```python
from build123d import *

# Parameters (mm, degrees)
SKETCH1_R           = 1.6
BOSS_EXTRUDE1_DEPTH = 27
CUT_EXTRUDE1_REACH  = 138.335
SKETCH2_R           = 2.1
CUT_EXTRUDE2_REACH  = 155.174
SKETCH3_R           = 1.7
SKETCH3_3_R         = 3
SKETCH3_3_R_2       = 1.7
CUT_EXTRUDE3_DEPTH  = 3
SKETCH4_R           = 3
CUT_EXTRUDE4_DEPTH  = 8
BOSS_EXTRUDE2_START = -27
BOSS_EXTRUDE2_DEPTH = 27
FILLET1_R           = 10


with BuildPart() as part:
    # Sketch1 → Boss-Extrude1 (new body)
    with BuildSketch(Plane.XY.offset(10)):
        with BuildLine():
            Line((-25.534872354, -37.053613776), (50.619597549, -89.534180987))
            ThreePointArc((50.619597549, -89.534180987), (54.361803385, -90.334528675), (57.573873786, -88.254320829))
            Line((57.573873786, -88.254320829), (58.227827632, -87.305369414))
            ThreePointArc((58.227827632, -87.305369414), (59.02817532, -83.563163578), (56.947967474, -80.351093178))
            Line((56.947967474, -80.351093178), (-21.854778729, -26.045511066))
            ThreePointArc((-21.854778729, -26.045511066), (-26.045511066, 21.854778729), (21.854778729, 26.045511066))
            Line((21.854778729, 26.045511066), (89.019290298, -42.129978983))
            ThreePointArc((89.019290298, -42.129978983), (92.543786433, -43.620813626), (96.090160837, -42.182797794))
            Line((96.090160837, -42.182797794), (96.911137653, -41.373995292))
            ThreePointArc((96.911137653, -41.373995292), (98.401972296, -37.849499157), (96.963956464, -34.303124754))
            Line((96.963956464, -34.303124754), (32.056602073, 31.581232775))
            ThreePointArc((32.056602073, 31.581232775), (-34.47199994, 28.925442436), (-25.534872354, -37.053613776))
        make_face()
        with Locations((90.17973297, -37.494440018)):
            Circle(SKETCH1_R, mode=Mode.SUBTRACT)
        with Locations((68.973861607, -16.273907044)):
            Circle(SKETCH1_R, mode=Mode.SUBTRACT)
        with Locations((47.767990244, 4.946625931)):
            Circle(SKETCH1_R, mode=Mode.SUBTRACT)
        with Locations((18.75, 32.475952642)):
            Circle(SKETCH1_R, mode=Mode.SUBTRACT)
        with Locations((-6.511806663, 36.930290738)):
            Circle(SKETCH1_R, mode=Mode.SUBTRACT)
        with Locations((-28.726666617, 24.104535363)):
            Circle(SKETCH1_R, mode=Mode.SUBTRACT)
        with Locations((-37.5, 0)):
            Circle(SKETCH1_R, mode=Mode.SUBTRACT)
        with Locations((-28.726666617, -24.104535363)):
            Circle(SKETCH1_R, mode=Mode.SUBTRACT)
        with Locations((3.423348889, -47.901259716)):
            Circle(SKETCH1_R, mode=Mode.SUBTRACT)
        with Locations((28.003855203, -65.100059364)):
            Circle(SKETCH1_R, mode=Mode.SUBTRACT)
        with Locations((52.584361518, -82.298859012)):
            Circle(SKETCH1_R, mode=Mode.SUBTRACT)
    extrude(amount=BOSS_EXTRUDE1_DEPTH)

    # Sketch2 → Cut-Extrude1 (cut, up to next)
    with BuildSketch(Plane.XY.offset(37), mode=Mode.PRIVATE) as cut_extrude1_sk1:
        with Locations((52.584361518, -82.298859012)):
            Circle(SKETCH2_R)
    cut_extrude1_tool1 = extrude(cut_extrude1_sk1.sketch, amount=-CUT_EXTRUDE1_REACH, mode=Mode.PRIVATE) & part.part
    # Sketch2 → Cut-Extrude1 (cut, up to next)
    with BuildSketch(Plane.XY.offset(37), mode=Mode.PRIVATE) as cut_extrude1_sk2:
        with Locations((28.003855203, -65.100059364)):
            Circle(SKETCH2_R)
    cut_extrude1_tool2 = extrude(cut_extrude1_sk2.sketch, amount=-CUT_EXTRUDE1_REACH, mode=Mode.PRIVATE) & part.part
    # Sketch2 → Cut-Extrude1 (cut, up to next)
    with BuildSketch(Plane.XY.offset(37), mode=Mode.PRIVATE) as cut_extrude1_sk3:
        with Locations((3.423348889, -47.901259716)):
            Circle(SKETCH2_R)
    cut_extrude1_tool3 = extrude(cut_extrude1_sk3.sketch, amount=-CUT_EXTRUDE1_REACH, mode=Mode.PRIVATE) & part.part
    # Sketch2 → Cut-Extrude1 (cut, up to next)
    with BuildSketch(Plane.XY.offset(37), mode=Mode.PRIVATE) as cut_extrude1_sk4:
        with Locations((-28.726666617, -24.104535363)):
            Circle(SKETCH2_R)
    cut_extrude1_tool4 = extrude(cut_extrude1_sk4.sketch, amount=-CUT_EXTRUDE1_REACH, mode=Mode.PRIVATE) & part.part
    # Sketch2 → Cut-Extrude1 (cut, up to next)
    with BuildSketch(Plane.XY.offset(37), mode=Mode.PRIVATE) as cut_extrude1_sk5:
        with Locations((-37.5, 0)):
            Circle(SKETCH2_R)
    cut_extrude1_tool5 = extrude(cut_extrude1_sk5.sketch, amount=-CUT_EXTRUDE1_REACH, mode=Mode.PRIVATE) & part.part
    # Sketch2 → Cut-Extrude1 (cut, up to next)
    with BuildSketch(Plane.XY.offset(37), mode=Mode.PRIVATE) as cut_extrude1_sk6:
        with Locations((-28.726666617, 24.104535363)):
            Circle(SKETCH2_R)
    cut_extrude1_tool6 = extrude(cut_extrude1_sk6.sketch, amount=-CUT_EXTRUDE1_REACH, mode=Mode.PRIVATE) & part.part
    # Sketch2 → Cut-Extrude1 (cut, up to next)
    with BuildSketch(Plane.XY.offset(37), mode=Mode.PRIVATE) as cut_extrude1_sk7:
        with Locations((-6.511806663, 36.930290738)):
            Circle(SKETCH2_R)
    cut_extrude1_tool7 = extrude(cut_extrude1_sk7.sketch, amount=-CUT_EXTRUDE1_REACH, mode=Mode.PRIVATE) & part.part
    # Sketch2 → Cut-Extrude1 (cut, up to next)
    with BuildSketch(Plane.XY.offset(37), mode=Mode.PRIVATE) as cut_extrude1_sk8:
        with Locations((18.75, 32.475952642)):
            Circle(SKETCH2_R)
    cut_extrude1_tool8 = extrude(cut_extrude1_sk8.sketch, amount=-CUT_EXTRUDE1_REACH, mode=Mode.PRIVATE) & part.part
    # Sketch2 → Cut-Extrude1 (cut, up to next)
    with BuildSketch(Plane.XY.offset(37), mode=Mode.PRIVATE) as cut_extrude1_sk9:
        with Locations((47.767990244, 4.946625931)):
            Circle(SKETCH2_R)
    cut_extrude1_tool9 = extrude(cut_extrude1_sk9.sketch, amount=-CUT_EXTRUDE1_REACH, mode=Mode.PRIVATE) & part.part
    # Sketch2 → Cut-Extrude1 (cut, up to next)
    with BuildSketch(Plane.XY.offset(37), mode=Mode.PRIVATE) as cut_extrude1_sk10:
        with Locations((68.973861607, -16.273907044)):
            Circle(SKETCH2_R)
    cut_extrude1_tool10 = extrude(cut_extrude1_sk10.sketch, amount=-CUT_EXTRUDE1_REACH, mode=Mode.PRIVATE) & part.part
    # Sketch2 → Cut-Extrude1 (cut, up to next)
    with BuildSketch(Plane.XY.offset(37), mode=Mode.PRIVATE) as cut_extrude1_sk11:
        with Locations((90.17973297, -37.494440018)):
            Circle(SKETCH2_R)
    cut_extrude1_tool11 = extrude(cut_extrude1_sk11.sketch, amount=-CUT_EXTRUDE1_REACH, mode=Mode.PRIVATE) & part.part
    add(cut_extrude1_tool1.solids().sort_by_distance((52.584362, -82.298859, 37))[0], mode=Mode.SUBTRACT)
    add(cut_extrude1_tool2.solids().sort_by_distance((28.003855, -65.100059, 37))[0], mode=Mode.SUBTRACT)
    add(cut_extrude1_tool3.solids().sort_by_distance((3.423349, -47.90126, 37))[0], mode=Mode.SUBTRACT)
    add(cut_extrude1_tool4.solids().sort_by_distance((-28.726667, -24.104535, 37))[0], mode=Mode.SUBTRACT)
    add(cut_extrude1_tool5.solids().sort_by_distance((-37.5, 0, 37))[0], mode=Mode.SUBTRACT)
    add(cut_extrude1_tool6.solids().sort_by_distance((-28.726667, 24.104535, 37))[0], mode=Mode.SUBTRACT)
    add(cut_extrude1_tool7.solids().sort_by_distance((-6.511807, 36.930291, 37))[0], mode=Mode.SUBTRACT)
    add(cut_extrude1_tool8.solids().sort_by_distance((18.75, 32.475953, 37))[0], mode=Mode.SUBTRACT)
    add(cut_extrude1_tool9.solids().sort_by_distance((47.76799, 4.946626, 37))[0], mode=Mode.SUBTRACT)
    add(cut_extrude1_tool10.solids().sort_by_distance((68.973862, -16.273907, 37))[0], mode=Mode.SUBTRACT)
    add(cut_extrude1_tool11.solids().sort_by_distance((90.179733, -37.49444, 37))[0], mode=Mode.SUBTRACT)

    # Sketch3 → Cut-Extrude2 (cut, up to next)
    with BuildSketch(Plane(origin=(-25.534872354, -37.053613776, 0), x_dir=(0.823413639467006, -0.567441607867893, 0), z_dir=(-0.5674416078678929, -0.8234136394670059, 0)), mode=Mode.PRIVATE) as cut_extrude2_sk1:
        with Locations((15, 23.5)):
            Circle(SKETCH3_R)
    cut_extrude2_tool1 = extrude(cut_extrude2_sk1.sketch, amount=-CUT_EXTRUDE2_REACH, mode=Mode.PRIVATE) & part.part
    add(cut_extrude2_tool1.solids().sort_by_distance((-13.183668, -45.565238, 23.5))[0], mode=Mode.SUBTRACT)

    # Sketch3<3> → Cut-Extrude3 (cut)
    with BuildSketch(Plane(origin=(-25.534872354, -37.053613776, 0), x_dir=(0.823413639467006, -0.567441607867893, 0), z_dir=(-0.5674416078678929, -0.8234136394670059, 0))):
        with Locations((15, 23.5)):
            Circle(SKETCH3_3_R)
        with Locations((15, 23.5)):
            Circle(SKETCH3_3_R_2, mode=Mode.SUBTRACT)
    extrude(amount=-CUT_EXTRUDE3_DEPTH, mode=Mode.SUBTRACT)

    # Sketch4 → Cut-Extrude4 (cut)
    with BuildSketch(Plane.XY.offset(37)):
        with Locations((18.75, 32.475952642)):
            Circle(SKETCH4_R)
        with Locations((-28.726666617, 24.104535363)):
            Circle(SKETCH4_R)
        with Locations((-28.726666617, -24.104535363)):
            Circle(SKETCH4_R)
    cut_extrude4 = extrude(amount=-CUT_EXTRUDE4_DEPTH, mode=Mode.SUBTRACT)

    # Sketch5 → Boss-Extrude2 (add)
    with BuildSketch(Plane.XY.offset(37).offset(BOSS_EXTRUDE2_START)):
        with BuildLine():
            Line((-19.283628291, -22.981333294), (-21.854778729, -26.045511066))
            ThreePointArc((-21.854778729, -26.045511066), (-26.045511066, 21.854778729), (21.854778729, 26.045511066))
            Line((21.854778729, 26.045511066), (19.283628291, 22.981333294))
            ThreePointArc((19.283628291, 22.981333294), (-22.981333294, 19.283628291), (-19.283628291, -22.981333294))
        make_face()
    extrude(amount=BOSS_EXTRUDE2_DEPTH)

    # Fillet1
    # the kernel refuses this fillet: 10 mm, written as the material it takes off along each edge
    with BuildSketch(Plane(origin=(-19.283628291, -22.981333294, -6.269784336), x_dir=(-0.6427876096873701, -0.7660444431182809, 0), z_dir=(0, 0, 1))) as fillet1_piece_1:
        with BuildLine():
            CenterArc((9.058823529, -8.626024838), FILLET1_R, 120.389942449, 47.156356956)
            Line((-0.705882353, -6.469518628), (-0.901176471, -6.426388504))
            ThreePointArc((-0.901176471, -6.426388504), (-0.375812744, -3.232263822), (-0.2, 0))
            Line((-0.2, 0), (0, 0.2))
            ThreePointArc((0, 0.2), (2, 0.2), (3.898823529, 0.172520497))
            Line((3.898823529, 0.172520497), (4, 0))
        make_face()
    extrude(amount=59.539568673, mode=Mode.SUBTRACT)
    with BuildSketch(Plane(origin=(19.283628291, 22.981333294, -6.269784336), x_dir=(0.6427876096857099, 0.7660444431196739, 0), z_dir=(0, 0, 1))) as fillet1_piece_2:
        with BuildLine():
            CenterArc((9.058823529, 8.626024838), FILLET1_R, 192.453700594, 47.156356956)
            Line((-0.705882353, 6.469518628), (-0.901176471, 6.426388504))
            ThreePointArc((-0.901176471, 6.426388504), (-0.375812744, 3.232263822), (-0.2, 0))
            Line((-0.2, 0), (0, -0.2))
            ThreePointArc((0, -0.2), (2, -0.2), (3.898823529, -0.172520497))
            Line((3.898823529, -0.172520497), (4, 0))
        make_face()
    extrude(amount=59.539568673, mode=Mode.SUBTRACT)

    # Mirror1: Cut-Extrude4 across plane
    add(cut_extrude4.mirror(Plane.XY.offset(23.5)), mode=Mode.SUBTRACT)


solid = part.part
```
Verification items for the finished model (mm, model axes). A direction names the side the tool comes from. Give positions to 0.01 mm unless a question says otherwise; leave off trailing zeros. Order: outer loops, then holes, each group sorted by start corner. A loop starts at its lowest first (then second) coordinate and runs counter-clockwise, first axis right, second up. Notation, with made-up numbers: (13.25, 53) -> (65.25, 53) arc R21 ccw to (65.25, 81) -> close; hole circle Ø2 at (29, -35.5). An arc over 180 degrees is marked (long way). One line per item, written item: value.
(1) Sectioned sample at A-A on y = 13. Record the cut outline in (x, z), then the cut area to 3 significant figures.
Final values:
outline: (-43.08, 10) -> (-27.04, 10) -> (-27.04, 37) -> (-43.08, 37) -> close; (34.71, 10) -> (50.36, 10) -> (50.36, 37) -> (34.71, 37) -> close
area: 856 mm^2
(2) Sectioned sample at B-B on x = 42.5. Record the cut outline in (y, z), then the cut area to 3 significant figures.
Final values:
outline: (-83.94, 10) -> (-70.39, 10) -> (-70.39, 37) -> (-83.94, 37) -> close; (5.09, 10) -> (20.98, 10) -> (20.98, 37) -> (5.09, 37) -> close
area: 795 mm^2
(3) Scan lines: line 1 along Y through (x, z) = (49, 18.75); line 2 along Y through (x, z) = (19.5, 36); line 3 along X through (y, z) = (4, 19.75). Record each from-to range of solid material in increasing order. Write a range as [from, to].
Final values:
line 1: [-88.42, -74.87], [-1.51, 3.25], [6.65, 14.38]
line 2: [-68.09, -54.54], [25.52, 29.57], [35.38, 40.56]
line 3: [-44.82, -29.73], [43.57, 45.89], [49.64, 59.23]
(4) Sectioned sample at C-C on x = 18.75. Record the cut outline in (y, z).
Final values:
outline: (-67.57, 10) -> (-54.03, 10) -> (-54.03, 37) -> (-67.57, 37) -> close; (25.47, 10) -> (29.48, 10) -> (29.48, 18) -> (30.38, 18) -> (30.38, 29) -> (29.48, 29) -> (29.48, 37) -> (25.47, 37) -> close; (34.58, 18) -> (35.48, 18) -> (35.48, 10) -> (40.91, 10) -> (40.91, 37) -> (35.48, 37) -> (35.48, 29) -> (34.58, 29) -> close
(5) Sectioned sample at D-D on y = -59. Record the cut outline in (x, z), then the cut area to 3 significant figures.
Final values:
outline: (6.31, 10) -> (25.97, 10) -> (25.97, 37) -> (6.31, 37) -> close
area: 531 mm^2
(6) Tool access check on faces 1 (the face through (19, 35, 29)), 2 (the face through (54.308, -90.344, 23.311)), 3 (the face through (17.749, 25.494, 23.311)), 4 (the face through (-9.869, -44.206, 23.542)). Record the directions out of +Z, -Z, +X, -X, +Y, -Y that give a thin tool (end or side, any length) a straight path to the whole face; none if there is none.
Final values:
face 1: +Z
face 2: +Z, -Z, -Y
face 3: +Z, -Z
face 4: none
(7) Draft check along Y on faces 5 (the face through (64.96, -1.82, 23.31)), 6 (the face through (-10, -37, 10)), 7 (the face through (55, -7.6, 23.3)), 8 (the face through (12.009, -62.927, 23.311)). Enter one of: pulls with the +Y half, pulls with the -Y half, needs draft (parallel to the pull), parting line crosses it, or undercut.
Final values:
face 5: pulls with the +Y half
face 6: needs draft
face 7: undercut
face 8: pulls with the -Y half
(8) Gauge pin test, flat ends, axial feed: pin 1 (8 mm diameter, centred on x = 22, z = 28.5, fed in from +Y); pin 2 (12 mm diameter, centred on y = -17.5, z = 30.5, fed in from -X); pin 3 (7 mm diameter, centred on x = -28.73, y = -24.1, fed in from +Z); pin 4 (6 mm diameter, centred on y = -72.5, z = 12.5, fed in from -X). Record the tip position at first contact, or that the pin passes through.
Final values:
pin 1: y = 41.24
pin 2: x = -43.51
pin 3: z = 37
pin 4: x = 21.55
